```python
from build123d import *

# Parameters (mm, degrees)
SKETCH1_W           = 138
SKETCH1_H           = 88
BOSS_EXTRUDE1_DEPTH = 3.81
CHAMFER1_SIZE       = 0.889
SKETCH2_W           = 128.222
SKETCH2_H           = 78.222
BOSS_EXTRUDE2_DEPTH = 5
SKETCH3_W           = 18
SKETCH3_H           = 18
CUT_EXTRUDE1_DEPTH  = 10
SKETCH4_W           = 18
SKETCH4_H           = 2
BOSS_EXTRUDE3_DEPTH = 3


with BuildPart() as part:
    # Sketch1 → Boss-Extrude1 (new body)
    with BuildSketch(Plane(origin=(0, 0, 0), x_dir=(1, 0, 0), z_dir=(0, 1, 0))):
        with Locations((32.17, -15.806)):
            Rectangle(SKETCH1_W, SKETCH1_H)
    extrude(amount=-BOSS_EXTRUDE1_DEPTH)

    # Chamfer1
    chamfer1_edges = [part.edges().sort_by_distance(p)[0] for p in [
        (-36.83, -3.81, 15.806),
        (32.17, -3.81, 59.806),
        (101.17, -3.81, 15.806),
        (32.17, 0, 59.806),
        (-36.83, 0, 15.806),
        (32.17, 0, -28.194),
        (101.17, 0, 15.806),
        (32.17, -3.81, -28.194),
        (101.17, -1.905, 59.806),
        (-36.83, -1.905, 59.806),
        (-36.83, -1.905, -28.194),
        (101.17, -1.905, -28.194),
    ]]
    chamfer(chamfer1_edges, length=CHAMFER1_SIZE)


with BuildPart() as body_2:
    # Sketch2 → Boss-Extrude2 (new body)
    with BuildSketch(Plane(origin=(0, -3.81, 0), x_dir=(1, 0, 0), z_dir=(0, 1, 0))):
        with Locations((32.17, -15.806)):
            Rectangle(SKETCH2_W, SKETCH2_H)
    extrude(amount=-BOSS_EXTRUDE2_DEPTH)


with BuildPart() as cut_extrude1_tool:
    # Sketch3 → Cut-Extrude1 (new body)
    with BuildSketch(Plane(origin=(0, 0, 0), x_dir=(-1, 0, 0), z_dir=(0, -1, 0))):
        with Locations((-1.599154352, -26.272344334)):
            Rectangle(SKETCH3_W, SKETCH3_H)
    extrude(amount=CUT_EXTRUDE1_DEPTH)


with BuildPart() as part_1:
    add(part.part)

    # Cut-Extrude1: cut by cut_extrude1_tool
    add(cut_extrude1_tool.part, mode=Mode.SUBTRACT)



with BuildPart() as body_2_1:
    add(body_2.part)

    # Cut-Extrude1: cut by cut_extrude1_tool
    add(cut_extrude1_tool.part, mode=Mode.SUBTRACT)


with BuildPart() as part_2:
    add(part_1.part)

    add(body_2_1.part)  # Boss-Extrude3 merges body 2
    # Sketch4 → Boss-Extrude3 (add)
    with BuildSketch(Plane(origin=(0, -3.81, 0), x_dir=(-1, 0, 0), z_dir=(0, -1, 0))):
        with Locations((-1.599154352, -18.272344334)):
            Rectangle(SKETCH4_W, SKETCH4_H)
        with Locations((-1.599154352, -34.272344334)):
            Rectangle(SKETCH4_W, SKETCH4_H)
    extrude(amount=BOSS_EXTRUDE3_DEPTH)


solid = part_2.part
```
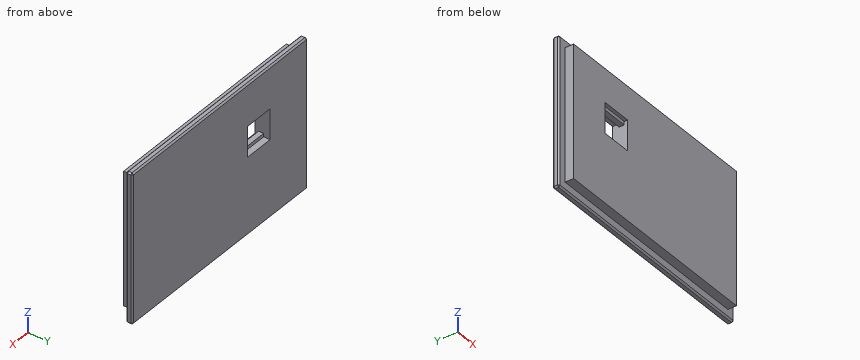
The model under review builds one solid part; all positions refer to its coordinate system, in mm. Give positions to 0.01 mm unless a question says otherwise; leave off trailing zeros. Order: outer loops, then holes, each group sorted by start corner. A loop starts at its lowest first (then second) coordinate and runs counter-clockwise, first axis right, second up. Notation, with made-up numbers: (47, -20) - (87, -20) arc R6 cw to (87, -9) - close; hole circle Ø11 at (-13.75, 76). An arc over 180 degrees is marked (long way). Use CSV: the item, a comma, the result in double quotes. Start each with the question number.
Q1. Clearance check with flat-ended pins moving along their axes: pin 1 Ø0.6 at (x, z) = (0.5, 34) entering from +Y; pin 2 Ø1 at (x, y) = (-14.5, -8) entering from +Z; pin 3 Ø3 at (y, z) = (-4.5, 20) entering from -X. State where each tip first meets the part, or that it passes through.
Q2. We need section D-D, the plane x = 92. Write out the cut boundary in (y, z) (3 decimals), and give its area (3 significant figures).
Q3. We need section C-C, the plane z = 43. Write out the cut boundary in (x, y), and give its area (3 significant figures).
Q4. We need section A-A, the plane z = 22. Write out the cut boundary in (x, y).
Q5. To check wall thickness, follow line 1 along Z through (x, y) = (6.5, -7.5) (3 decimals); line 2 along Z through (x, y) = (11.5, -5.5) (3 decimals); line 3 along X through (y, z) = (-5.5, 8.5). State the ranges of each line that lie inside material, in increasing order. Write a range as [from, to].
Q6. We need section B-B, the plane x = -2.5. Write out the cut boundary in (y, z) (3 decimals).
Outcome:
1,pin 1,"stops at y = -3.81"
1,pin 2,"stops at z = 54.92"
1,pin 3,"stops at x = -36.75"
2,outline,"(-8.81, -23.305) - (-3.81, -23.305) - (-3.81, -27.305) - (-2.921, -28.194) - (-0.889, -28.194) - (0, -27.305) - (0, 58.917) - (-0.889, 59.806) - (-2.921, 59.806) - (-3.81, 58.917) - (-3.81, 54.917) - (-8.81, 54.917) - close"
2,area,"725 mm^2"
3,outline,"(-36.83, -2.92) - (-35.94, -3.81) - (-31.94, -3.81) - (-31.94, -8.81) - (96.28, -8.81) - (96.28, -3.81) - (100.28, -3.81) - (101.17, -2.92) - (101.17, -0.89) - (100.28, 0) - (-35.94, 0) - (-36.83, -0.89) - close"
3,area,"1,170 mm^2"
4,outline,"(-36.83, -2.92) - (-35.94, -3.81) - (-31.94, -3.81) - (-31.94, -8.81) - (-7.4, -8.81) - (-7.4, 0) - (-35.94, 0) - (-36.83, -0.89) - close; (10.6, -8.81) - (96.28, -8.81) - (96.28, -3.81) - (100.28, -3.81) - (101.17, -2.92) - (101.17, -0.89) - (100.28, 0) - (10.6, 0) - close"
5,line 1,"z = [-23.305, 17.272], [35.272, 54.917]"
5,line 2,"z = [-23.305, 54.917]"
5,line 3,"x = [-31.94, 96.28]"
6,outline,"(-8.81, -23.305) - (-3.81, -23.305) - (-3.81, -27.305) - (-2.921, -28.194) - (-0.889, -28.194) - (0, -27.305) - (0, 17.272) - (-3.81, 17.272) - (-3.81, 19.272) - (-6.81, 19.272) - (-6.81, 17.272) - (-8.81, 17.272) - close; (-8.81, 35.272) - (-6.81, 35.272) - (-6.81, 33.272) - (-3.81, 33.272) - (-3.81, 35.272) - (0, 35.272) - (0, 58.917) - (-0.889, 59.806) - (-2.921, 59.806) - (-3.81, 58.917) - (-3.81, 54.917) - (-8.81, 54.917) - close"
